Build history of the part. All positions in model axes, mm. A direction names the side the tool comes from. Give positions to 0.01 mm unless a question says otherwise; leave off trailing zeros. Order: outer loops, then holes, each group sorted by start corner. A loop starts at its lowest first (then second) coordinate and runs counter-clockwise, first axis right, second up. Notation, with made-up numbers: (64.5, 14) -> (103.5, 14) arc R17 ccw to (103.5, 42) -> close; hole circle Ø8 at (70.5, -22.5). An arc over 180 degrees is marked (long way). One line per item, written item: value. Start each with the question number.
(1) Two-plate mould, pull along X, no slides. Class faces 6 (the flat face through (43, 6.3, -2)), 7 (the flat face through (51.958, 15.782, -5.916)): +X half, -X half, draft (parallel to the pull), parting line (faces both ways), or undercut.
(2) Saw through at B-B on x = -4. Give the cut face in (y, z).
(3) Pin check, flat tips, straight feed: pin 1 (4 mm diameter, centred on y = 46.5, z = -10.5, fed in from +X); pin 2 (1 mm diameter, centred on x = 15.5, z = -4, fed in from +Y); pin 3 (0.5 mm diameter, centred on x = 63, z = -7, fed in from +Y). Stop position of each tip, or through.
(4) Which spindle directions (+Z, -Z, +X, -X, +Y, -Y) get a long thin tool onto all of the face, cutting with end or side? Do faces 1 (the cylindrical face through (-7.81, 22.99, -5.92)), 2 (the flat face through (-10, 51.3, -8)), 3 (the flat face through (43, 5, -3.6)), 4 (the flat face through (43.375, 1.584, -1.84)), 5 (the flat face through (86.3, 15.7, -5.9)). Say none if no direction does.
(5) Probe line 1 (Y direction, x = 13, z = -4.25); line 2 (Y direction, x = -6, z = -8.5); line 3 (Y direction, x = -15, z = -10.5). List the from-to ranges inside material, lowest first.
(6) Saw through at A-A on y = 42. Give the cut face in (x, z).
```python
from build123d import *

# Parameters (mm, degrees)
BLANKSKE_W          = 105
BLANKSKE_H          = 18
BLANK_DEPTH         = 12
TOOTHCUTSIM_DEPTH   = 108.205410311
TEETHCUTS_COUNT     = 18
TEETHCUTS_PITCH     = 6.2831853
CUT_EXTRUDE1_DEPTH  = 108.205410311
BOSS_EXTRUDE1_DEPTH = 20
FILLET2_R           = 7
CUT_EXTRUDE2_DEPTH  = 9
CUT_EXTRUDE3_DEPTH  = 3
CUT_EXTRUDE4_REACH  = 122.698
SKETCH5_R           = 2


with BuildPart() as part:
    # BlankSke → Blank (new body)
    with BuildSketch(Plane.XY):
        with Locations((52.5, 9)):
            Rectangle(BLANKSKE_W, BLANKSKE_H)
    extrude(amount=-BLANK_DEPTH)

    # TooCutSkeSim → ToothCutSim (cut, through all)
    with BuildSketch(Plane.XY):
        Polygon((0.861870739, 13.5), (-0.861870739, 13.5), (-2.508981637, 18.0254), (2.508981637, 18.0254), align=None)
    toothcutsim = extrude(amount=-TOOTHCUTSIM_DEPTH, mode=Mode.SUBTRACT)

    # TeethCuts: ToothCutSim ×18
    with Locations(*[(i * TEETHCUTS_PITCH, 0, 0) for i in range(1, TEETHCUTS_COUNT)]):
        add(toothcutsim, mode=Mode.SUBTRACT)

    # Sketch1 → Cut-Extrude1 (cut, through all)
    with BuildSketch(Plane(origin=(105, 0, 0), x_dir=(0, 0, -1), z_dir=(1, 0, 0))):
        Polygon((0, 0), (3.424264069, 0), (0.3, 3.124264069), (0.3, 3.7), (3.6, 3.7), (3.6, 6.3), (0, 6.3), align=None)
        Polygon((11.7, 3.124264069), (8.575735931, 0), (12, 0), (12, 6.3), (8.4, 6.3), (8.4, 3.7), (11.7, 3.7), align=None)
    extrude(amount=-CUT_EXTRUDE1_DEPTH, mode=Mode.SUBTRACT)

    # Sketch2 → Boss-Extrude1 (add)
    with BuildSketch(Plane.ZY):
        Polygon((-12, 58.3), (0, 58.3), (0, 6.3), (-3.6, 6.3), (-3.6, 3.7), (-0.3, 3.7), (-0.3, 3.124264069), (-3.424264069, 0), (-8.575735931, 0), (-11.7, 3.124264069), (-11.7, 3.7), (-8.4, 3.7), (-8.4, 6.3), (-12, 6.3), align=None)
    extrude(amount=BOSS_EXTRUDE1_DEPTH)

    # Fillet2
    fillet2_edges = [part.edges().sort_by_distance(p)[0] for p in [
        (0, 58.3, -6),
        (-20, 58.3, -6),
    ]]
    fillet(fillet2_edges, radius=FILLET2_R)

    # Sketch3 → Cut-Extrude2 (cut)
    with BuildSketch(Plane(origin=(0, 58.3, 0), x_dir=(1, 0, 0), z_dir=(0, 1, 0))):
        with BuildLine():
            ThreePointArc((-8.5, 6), (-8.939339828, 7.060660172), (-10, 7.5))
            Line((-10, 7.5), (-10, 4.5))
            ThreePointArc((-10, 4.5), (-8.939339828, 4.939339828), (-8.5, 6))
        make_face()
        with BuildLine():
            Line((-10, 4.5), (-10, 7.5))
            ThreePointArc((-10, 7.5), (-11.5, 6), (-10, 4.5))
        make_face()
    extrude(amount=-CUT_EXTRUDE2_DEPTH, mode=Mode.SUBTRACT)

    # Sketch4 → Cut-Extrude3 (cut)
    with BuildSketch(Plane(origin=(0, 54.3, 0), x_dir=(1, 0, 0), z_dir=(0, 1, 0))):
        Polygon((-13.05, 12), (-13.05, 7.760918321), (-13.05, 6), (-13.05, 4.239081679), (-11.525, 3.358622518), (-10, 2.478163358), (-8.475, 3.358622518), (-6.95, 4.239081679), (-6.95, 6), (-6.95, 7.760918321), (-6.95, 12), align=None)
        with BuildLine():
            ThreePointArc((-8.75, 6), (-10, 4.75), (-11.25, 6))
            ThreePointArc((-11.25, 6), (-10, 7.25), (-8.75, 6))
        make_face(mode=Mode.SUBTRACT)
    extrude(amount=-CUT_EXTRUDE3_DEPTH, mode=Mode.SUBTRACT)

    # Sketch5 → Cut-Extrude4 (cut, up to next)
    with BuildSketch(Plane.XY, mode=Mode.PRIVATE) as cut_extrude4_sk1:
        with Locations((-8.8817, 42)):
            Circle(SKETCH5_R)
    cut_extrude4_tool1 = extrude(cut_extrude4_sk1.sketch, amount=-CUT_EXTRUDE4_REACH, mode=Mode.PRIVATE) & part.part
    # Sketch5 → Cut-Extrude4 (cut, up to next)
    with BuildSketch(Plane.XY, mode=Mode.PRIVATE) as cut_extrude4_sk2:
        with Locations((-8.8817, 21.3)):
            Circle(SKETCH5_R)
    cut_extrude4_tool2 = extrude(cut_extrude4_sk2.sketch, amount=-CUT_EXTRUDE4_REACH, mode=Mode.PRIVATE) & part.part
    add(cut_extrude4_tool1.solids().sort_by_distance((-8.8817, 42, 0))[0], mode=Mode.SUBTRACT)
    add(cut_extrude4_tool2.solids().sort_by_distance((-8.8817, 21.3, 0))[0], mode=Mode.SUBTRACT)


solid = part.part
```
Results below:
1. face 6: draft
1. face 7: undercut
2. outline: (0, -8.58) -> (3.12, -11.7) -> (3.7, -11.7) -> (3.7, -8.4) -> (6.3, -8.4) -> (6.3, -12) -> (57.62, -12) -> (57.62, 0) -> (6.3, 0) -> (6.3, -3.6) -> (3.7, -3.6) -> (3.7, -0.3) -> (3.12, -0.3) -> (0, -3.42) -> close
3. pin 1: stops at x = 0
3. pin 2: stops at y = 18
3. pin 3: stops at y = 13.5
4. face 1: +Z, -Z
4. face 2: -Z
4. face 3: +Z, +X, -X
4. face 4: +Z, +X, -X, -Y
4. face 5: +Z, -Z, +Y
5. line 1: y = 0 to 13.5
5. line 2: y = 0 to 3.7, 6.3 to 58.23
5. line 3: y = 1.92 to 3.7, 6.3 to 58.01
6. outline: (-20, -12) -> (-10.88, -12) -> (-10.88, 0) -> (-20, 0) -> close; (-6.88, -12) -> (0, -12) -> (0, 0) -> (-6.88, 0) -> close
